Check sheet for the modelled part. Datum: model origin and axes. Units: mm. A direction names the side the tool comes from. Give positions to 0.01 mm unless a question says otherwise; leave off trailing zeros. Order: outer loops, then holes, each group sorted by start corner. A loop starts at its lowest first (then second) coordinate and runs counter-clockwise, first axis right, second up.
```python
from build123d import *

# Parameters (mm, degrees)
F1_DEPTH = 10
F2_DEPTH = 12
F3_SIZE  = 5
F4_SIZE  = 1.99999
F5_R     = 7.5
F6_DEPTH = 5
F7_R     = 4.99999
F9_DEPTH = 3


# Not quite as in the source:
# - a fillet or chamfer is up to 0.001 mm smaller than in the source, because OpenCascade refuses the exact size
# - a feature names something its author has since deleted; it is built from what else it names


with BuildPart() as f1:
    # F0 (on Right) → F1 (new body)
    with BuildSketch(Plane.YZ):
        with BuildLine():
            Line((11.25, 3.75), (20.2777587519, 9.75))
            ThreePointArc((20.2777587519, 9.75), (15.9099025767, 15.9099025767), (9.75, 20.2777587519))
            Line((9.75, 20.2777587519), (3.75, 11.25))
            Line((3.75, 11.25), (0, 11.25))
            Line((0, 11.25), (-3.75, 11.25))
            Line((-3.75, 11.25), (-9.75, 20.2777587519))
            ThreePointArc((-9.75, 20.2777587519), (-15.9099025767, 15.9099025767), (-20.2777587519, 9.75))
            Line((-20.2777587519, 9.75), (-11.25, 3.75))
            Line((-11.25, 3.75), (-11.25, 0))
            Line((-11.25, 0), (-11.25, -3.75))
            Line((-11.25, -3.75), (-20.2777587519, -9.75))
            ThreePointArc((-20.2777587519, -9.75), (-15.9099025767, -15.9099025767), (-9.75, -20.2777587519))
            Line((-9.75, -20.2777587519), (-3.75, -11.25))
            Line((-3.75, -11.25), (0, -11.25))
            Line((0, -11.25), (3.75, -11.25))
            Line((3.75, -11.25), (9.75, -20.2777587519))
            ThreePointArc((9.75, -20.2777587519), (15.9099025767, -15.9099025767), (20.2777587519, -9.75))
            Line((20.2777587519, -9.75), (11.25, -3.75))
            Line((11.25, -3.75), (11.25, 0))
            Line((11.25, 0), (11.25, 3.75))
        make_face()
    extrude(amount=F1_DEPTH)

    # F0 (on Right) → F2 (join)
    with BuildSketch(Plane.YZ):
        with BuildLine():
            Line((3.75, 11.25), (9.75, 20.2777587519))
            ThreePointArc((9.75, 20.2777587519), (0, 22.5), (-9.75, 20.2777587519))
            Line((-9.75, 20.2777587519), (-3.75, 11.25))
            Line((-3.75, 11.25), (0, 11.25))
            Line((0, 11.25), (3.75, 11.25))
        make_face()
        with BuildLine():
            ThreePointArc((-9.75, 20.2777587519), (0, 22.5), (9.75, 20.2777587519))
            Line((9.75, 20.2777587519), (6, 25.5))
            Line((6, 25.5), (0, 25.5))
            Line((0, 25.5), (-6, 25.5))
            Line((-6, 25.5), (-9.75, 20.2777587519))
        make_face()
        with BuildLine():
            Line((-11.25, 3.75), (-20.2777587519, 9.75))
            ThreePointArc((-20.2777587519, 9.75), (-22.5, 0), (-20.2777587519, -9.75))
            Line((-20.2777587519, -9.75), (-11.25, -3.75))
            Line((-11.25, -3.75), (-11.25, 0))
            Line((-11.25, 0), (-11.25, 3.75))
        make_face()
        with BuildLine():
            ThreePointArc((-20.2777587519, -9.75), (-22.5, 0), (-20.2777587519, 9.75))
            Line((-20.2777587519, 9.75), (-25.5, 6))
            Line((-25.5, 6), (-25.5, 0))
            Line((-25.5, 0), (-25.5, -6))
            Line((-25.5, -6), (-20.2777587519, -9.75))
        make_face()
        with BuildLine():
            ThreePointArc((-9.75, -20.2777587519), (0, -22.5), (9.75, -20.2777587519))
            Line((9.75, -20.2777587519), (3.75, -11.25))
            Line((3.75, -11.25), (0, -11.25))
            Line((0, -11.25), (-3.75, -11.25))
            Line((-3.75, -11.25), (-9.75, -20.2777587519))
        make_face()
        with BuildLine():
            Line((6, -25.5), (9.75, -20.2777587519))
            ThreePointArc((9.75, -20.2777587519), (0, -22.5), (-9.75, -20.2777587519))
            Line((-9.75, -20.2777587519), (-6, -25.5))
            Line((-6, -25.5), (0, -25.5))
            Line((0, -25.5), (6, -25.5))
        make_face()
        with BuildLine():
            ThreePointArc((20.2777587519, -9.75), (21.93740609, -5.0000214041), (22.5, 0))
            ThreePointArc((22.5, 0), (21.93740609, 5.0000214041), (20.2777587519, 9.75))
            Line((20.2777587519, 9.75), (11.25, 3.75))
            Line((11.25, 3.75), (11.25, 0))
            Line((11.25, 0), (11.25, -3.75))
            Line((11.25, -3.75), (20.2777587519, -9.75))
        make_face()
        with BuildLine():
            ThreePointArc((20.2777587519, 9.75), (21.93740609, 5.0000214041), (22.5, 0))
            ThreePointArc((22.5, 0), (21.93740609, -5.0000214041), (20.2777587519, -9.75))
            Line((20.2777587519, -9.75), (25.5, -6))
            Line((25.5, -6), (25.5, 0))
            Line((25.5, 0), (25.5, 6))
            Line((25.5, 6), (20.2777587519, 9.75))
        make_face()
    extrude(amount=F2_DEPTH)

    # F3
    f3_edges = [f1.edges().sort_by_distance(p)[0] for p in [
        (10, 15.909903, 15.909903),
        (10, -15.909903, 15.909903),
        (10, -15.909903, -15.909903),
        (10, 15.909903, -15.909903),
    ]]
    chamfer(f3_edges, length=F3_SIZE)

    # F4 (size 2 in the source; OpenCascade refuses exactly that, so slightly less here)
    f4_edges = [f1.edges().sort_by_distance(p)[0] for p in [
        (12, 0, 25.5),
        (12, -7.875, 22.888879),
        (12, 7.875, 22.888879),
        (12, -6.75, 15.763879),
        (12, 6.75, 15.763879),
        (12, 0, 11.25),
        (12, -15.763879, 6.75),
        (12, -22.888879, 7.875),
        (12, -25.5, 0),
        (12, -22.888879, -7.875),
        (12, -15.763879, -6.75),
        (12, -11.25, 0),
        (12, 0, -11.25),
        (12, -6.75, -15.763879),
        (12, -7.875, -22.888879),
        (12, 6.75, -15.763879),
        (12, 0, -25.5),
        (12, 7.875, -22.888879),
        (12, 15.763879, -6.75),
        (12, 11.25, 0),
        (12, 15.763879, 6.75),
        (12, 22.888879, 7.875),
        (12, 25.5, 0),
        (12, 22.888879, -7.875),
    ]]
    chamfer(f4_edges, length=F4_SIZE)

    # F5 (on face) → F6 (join)
    with BuildSketch(Plane.YZ.offset(10)):
        Circle(F5_R)
    extrude(amount=F6_DEPTH)

    # F7 (radius 5 in the source; OpenCascade refuses exactly that, so slightly less here)
    f7_edges = [f1.edges().sort_by_distance(p)[0] for p in [
        (15, -7.5, 0),
    ]]
    fillet(f7_edges, radius=F7_R)

    # F8 (on face) → F9 (cut)
    with BuildSketch(Plane.YZ):
        with BuildLine():
            ThreePointArc((0, -11.25), (7.9549512883, -7.9549512883), (11.25, 0))
            ThreePointArc((11.25, 0), (7.9549512883, 7.9549512883), (0, 11.25))
            ThreePointArc((0, 11.25), (-7.9549512883, 7.9549512883), (-11.25, 0))
            ThreePointArc((-11.25, 0), (-7.9549512883, -7.9549512883), (0, -11.25))
        make_face()
    extrude(amount=F9_DEPTH, mode=Mode.SUBTRACT)


solid = f1.part
```
(1) Material ranges on L1, parallel to Y at x = 10.25, z = -5.5; L2, parallel to X at y = -1, z = -19; L3, parallel to Z at x = 9.75, y = 8, recorded low to high.
Response values:
L1: y = -25.25 to -14.33, -5.09 to 5.09, 14.33 to 25.25
L2: x = 0 to 12
L3: z = -22.71 to -17.64, -15.84 to 15.84, 17.64 to 22.71
(2) Cross-section at A-A on x = 3.75. Enter the section's corners in (y, z).
Response values:
outline: (-25.5, -6) - (-20.28, -9.75) arc R22.5 ccw to (-9.75, -20.28) - (-6, -25.5) - (6, -25.5) - (9.75, -20.28) arc R22.5 ccw to (20.28, -9.75) - (25.5, -6) - (25.5, 6) - (20.28, 9.75) arc R22.5 ccw to (9.75, 20.28) - (6, 25.5) - (-6, 25.5) - (-9.75, 20.28) arc R22.5 ccw to (-20.28, 9.75) - (-25.5, 6) - close
(3) Gauge pin test, flat ends, axial feed: pin 1 Ø5 at (y, z) = (-17.5, -1) entering from +X; pin 2 Ø9.5 at (y, z) = (2, -8) entering from +X; pin 3 Ø8 at (y, z) = (-12.5, 10.5) entering from -X; pin 4 Ø3 at (x, z) = (3.5, 9.5) entering from -Y. Record the tip position at first contact, or that the pin passes through.
Response values:
pin 1: stops at x = 12
pin 2: stops at x = 14.9
pin 3: stops at x = 0
pin 4: stops at y = -22.71
(4) Set-up check for faces 4 (the face through (11.014, -5.948, 16.388)), 5 (the face through (12, 19, 0)), 6 (the face through (11.014, -16.388, -5.948)), 7 (the face through (8.229, -18.752, 8.736)): record each of +Z, -Z, +X, -X, +Y, -Y from which the full face is reachable in a straight line by a thin tool's end or side.
Response values:
face 4: +X, -Y
face 5: +Z, -Z, +X, +Y
face 6: -Z, +X
face 7: +Z, +X
(5) Release check for a two-part mould opening along Z. For faces 1 (the face through (11, -24.5, 0.1)), 2 (the face through (2.465, 15.985, 15.835)), 3 (the face through (11.01, 0.05, -12.26)) record: released by +Z, released by -Z, zero draft, split by the parting line, or undercut.
Response values:
face 1: zero draft
face 2: released by +Z
face 3: undercut
